Geometry check sheet. Reference: the model listing, model coordinates, mm. Face numbers are marked on the shaded views. A direction names the side the tool comes from. Coordinates: 2 decimals unless noted, no trailing zeros. Loops run counter-clockwise (first coordinate to the right, second up) from the corner with the lowest first, then second, coordinate; pieces in that order, holes last. Notation, with made-up numbers: (10.5, -21) - (46.5, -21) arc R22 ccw to (46.5, 18) - close; hole circle Ø3 at (85.25, 14). An arc over 180 degrees is marked (long way). One line per item, written item: value.
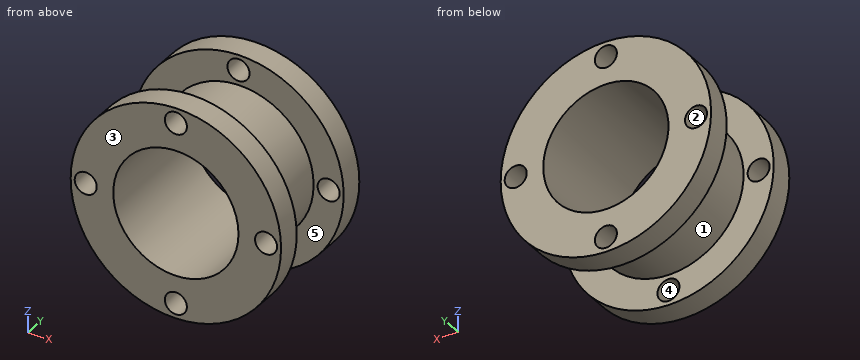
from build123d import *

# Parameters (mm, degrees)
F0_R     = 15
F0_R_2   = 12.5
F1_DEPTH = 25
F0_R_3   = 21
F3_DEPTH = 5
F4_R     = 21
F4_R_2   = 15
F5_DEPTH = 5
F6_D     = 4.4


# Not quite as in the source:
# - the program builds the solid bodies; features that only make, move or delete a surface that nothing else refers to are left out


with BuildPart() as f1:
    # F0 (on Front) → F1 (new body)
    with BuildSketch(Plane.XZ):
        Circle(F0_R)
        Circle(F0_R_2, mode=Mode.SUBTRACT)
    extrude(amount=F1_DEPTH)

    # F0 (on Front) → F3 (join)
    with BuildSketch(Plane.XZ):
        Circle(F0_R_3)
        Circle(F0_R, mode=Mode.SUBTRACT)
    extrude(amount=F3_DEPTH)

    # F4 (on face) → F5 (join)
    with BuildSketch(Plane.XZ.offset(25)):
        Circle(F4_R)
        Circle(F4_R_2, mode=Mode.SUBTRACT)
    extrude(amount=-F5_DEPTH)

    # F6 (through all)
    with Locations(Plane(origin=(0, 0, 0), x_dir=(1, 0, 0), z_dir=(0, 1, 0))):
        with Locations((-18, 0), (0, 18), (18, 0), (0, -18)):
            Hole(F6_D / 2)


solid = f1.part
(1) Cross-section at B-B on y = -2.75. Record the cut outline in (x, z).
Reply:
outline: circle Ø42 at (0, 0); hole circle Ø4.4 at (-18, 0); hole circle Ø25 at (0, 0); hole circle Ø4.4 at (0, -18); hole circle Ø4.4 at (0, 18); hole circle Ø4.4 at (18, 0)
(2) Cross-section at D-D on x = 18. Record the cut outline in (y, z), and give its area (3 significant figures).
Reply:
outline: (-25, -10.82) - (-20, -10.82) - (-20, -2.2) - (-25, -2.2) - close; (-25, 2.2) - (-20, 2.2) - (-20, 10.82) - (-25, 10.82) - close; (-5, -10.82) - (0, -10.82) - (0, -2.2) - (-5, -2.2) - close; (-5, 2.2) - (0, 2.2) - (0, 10.82) - (-5, 10.82) - close
area: 172 mm2
(3) Material ranges on probe 1 along Z at (x, y) = (0, -4.75); probe 2 along Y at (x, z) = (8, -15); probe 3 along Z at (x, y) = (-1, -4.75), recorded low to high. Write a range as from..to.
Reply:
probe 1: -21..-20.2, -15.8..-12.5, 12.5..15.8, 20.2..21
probe 2: -25..-20, -5..0
probe 3: -20.98..-19.96, -16.04..-12.46, 12.46..16.04, 19.96..20.98
(4) Go/stop test with flat-tipped pins: pin 1 Ø3 at (x, y) = (-16, -3.5) entering from +Z; pin 2 Ø10 at (y, z) = (-19.5, 5.5) entering from +X; pin 3 Ø10 at (x, y) = (1.5, -7) entering from -Z. Record where each tip stops, or that it passes through.
Reply:
pin 1: z = 15.19
pin 2: x = 20.99
pin 3: z = -21
(5) Cross-section at A-A on x = 0. State how many separate pieces and enclosed holes the cut face has, and give its area (3 significant figures).
Reply:
separate pieces: 6
enclosed holes: 0
area: 157 mm2
(6) Release check for a two-part mould opening along X. For the marked faces 1, 2 and 3 record: pulls with the +X half, pulls with the -X half, needs draft (parallel to the pull), parting line crosses it, or undercut.
Reply:
face 1: parting line crosses it
face 2: undercut
face 3: needs draft
(7) Access from +Z, -Z, +X, -X, +Y, -Y to the whole of each face (thin tool, end or side, straight path). Record for the marked faces 4 and 5.
Reply:
face 4: +Y, -Y
face 5: none
